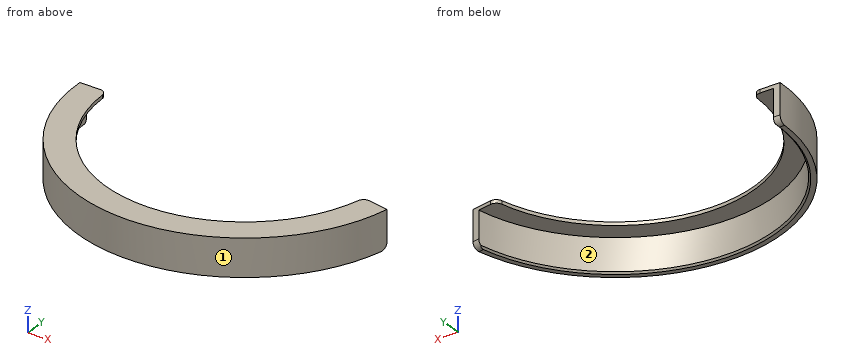
from build123d import *

# Parameters (mm, degrees)
F1_ANGLE = 170
F2_SIZE  = 0.5
F3_R     = 2


with BuildPart() as f1:
    # F0 (on Front) → F1 (revolve)
    with BuildSketch(Plane.XZ):
        Polygon((-49, 11), (-49, 0), (-47, 0), (-47, 10), (-41, 10), (-41, 11), align=None)
    revolve(axis=Axis((0, 0, 4.248688), (0, 0, 1)), revolution_arc=F1_ANGLE)

    # F2
    f2_edges = [f1.edges().sort_by_distance(p)[0] for p in [
        (-4.09632, -46.821151, 0),
    ]]
    chamfer(f2_edges, length=F2_SIZE)

    # F3
    f3_edges = [f1.edges().sort_by_distance(p)[0] for p in [
        (47.516974, -8.378525, 0),
        (-48.25, 0, 0),
        (-41, 0, 10.5),
        (40.377118, -7.119575, 10.5),
    ]]
    fillet(f3_edges, radius=F3_R)


solid = f1.part
Geometry: final body of the model. Coordinates: model frame, mm. Face numbers are marked on the shaded views. A direction names the side the tool comes from. Round coordinates to 2 decimals unless told otherwise and drop trailing zeros. Loops run counter-clockwise (first coordinate to the right, second up) from the corner with the lowest first, then second, coordinate; pieces in that order, holes last. Notation, with made-up numbers: (35, 57) -> (74, 57) arc R28 cw to (74, 94) -> close; hole circle Ø7 at (31.5, -38). An arc over 180 degrees is marked (long way). One line per question, with ' | ' between items. Start each with the question number.
1. Section B-B on z = 6.5. Output: boundary loops of the cut face in (x, y).
2. Contact query for flat-ended pins moving along their axis: pin 1 (1 mm diameter, centred on x = -7, z = 7.5, fed in from +Y); pin 2 (3 mm diameter, centred on y = -27, z = 2, fed in from +X); pin 3 (5 mm diameter, centred on x = -21, z = 7, fed in from +Y). Output: stop coordinate, or through.
3. Line query: line 1 along X through (y, z) = (-30, 2.25); line 2 along X through (y, z) = (-35.5, 8.25) (3 decimals); line 3 along Y through (x, z) = (0, 1.5). Output: solid intervals per line, ascending. Write a range as [from, to].
4. Section A-A on x = 0. Output: boundary loops of the cut face in (y, z), and give its area (3 significant figures).
5. Set-up query: the marked faces 1 and 2. Return all of +Z, -Z, +X, -X, +Y, -Y with unobstructed straight access to the full face (end or side cutting, diameter ignored); none if empty.
Returned:
1) outline: (-49, 0) arc R49 ccw to (48.26, -8.51) -> (46.29, -8.16) arc R47 cw to (-47, 0) -> close
2) pin 1: stops at y = -46.4 | pin 2: stops at x = 41.84 | pin 3: stops at y = -40.7
3) line 1: x = [-38.74, -36.18], [36.18, 38.74] | line 2: x = [-33.775, -30.802], [30.802, 33.775] | line 3: y = [-49, -47]
4) outline: (-49, 0) -> (-47.5, 0) -> (-47, 0.5) -> (-47, 10) -> (-41, 10) -> (-41, 11) -> (-49, 11) -> close | area: 27.9 mm2
5) face 1: +Z, -Z, -Y | face 2: -Z, +Y
